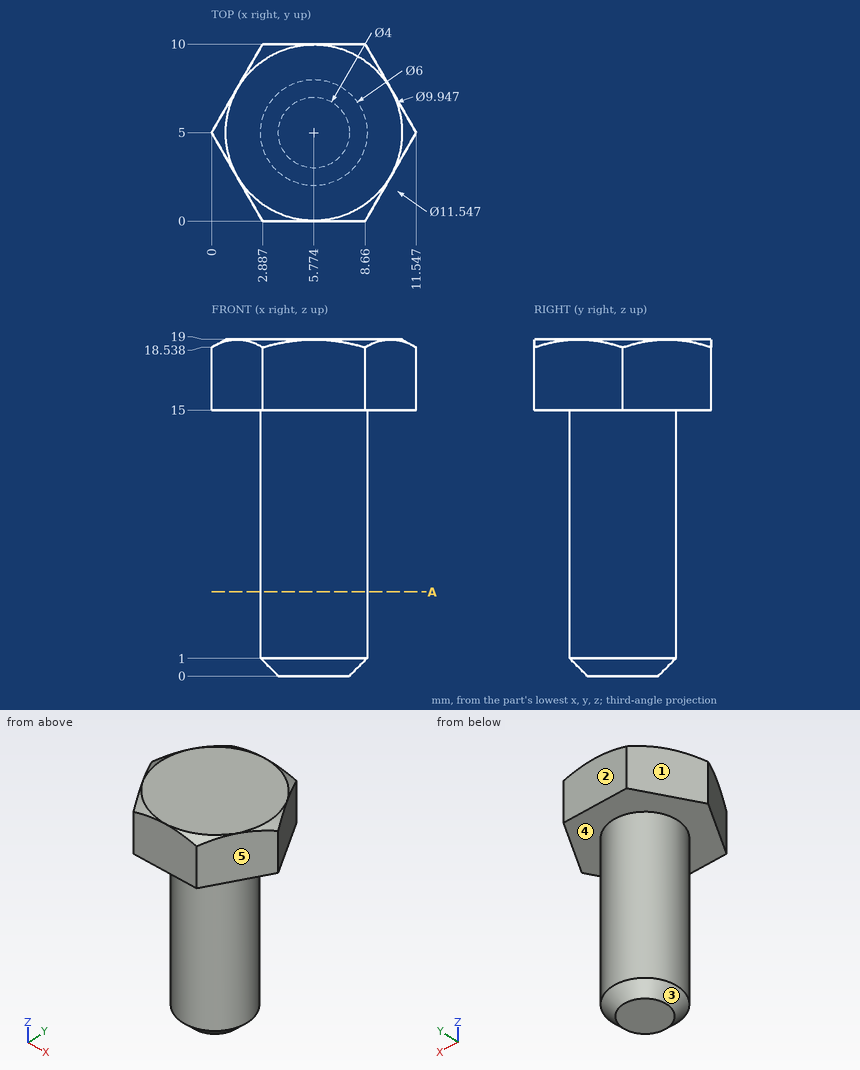
The figure shows three views and two pictorial views of one solid part (mm, origin at its lowest corner). Answer the questions. A direction names the side the tool comes from. Round coordinates to 2 decimals unless told otherwise and drop trailing zeros. Loops run counter-clockwise (first coordinate to the right, second up) from the corner with the lowest first, then second, coordinate; pieces in that order, holes last. Notation, with made-up numbers: M 85.5,-10 L 89.5,-10 A24 ccw 89.5,29 Z; hole C 14,70 d8. An arc over 180 degrees is marked long. Use CSV: the item, a comma, the result in double quotes.
Q1. Each of these flat-tipped pins is pushed along its axis until it touches: pin 1 (3 mm diameter, centred on y = 6, z = 3, fed in from -X); pin 2 (1 mm diameter, centred on y = 3.5, z = 8, fed in from -X) (1 decimal); pin 3 (5 mm diameter, centred on y = 7.5, z = 13.5, fed in from -X). Where does it stop, or does it pass through?
Determined:
pin 1,"x = 2.77"
pin 2,"x = 2.9"
pin 3,"x = 0.29"
Q2. A tool of negligible diameter and unlimited length cuts with its end or side. For the marked faces 4 and 5, from which of +Z, -Z, +X, -X, +Y, -Y can it reach the whole face along a straight path? Write none if from no direction.
Determined:
face 4,"-Z"
face 5,"+Z, -Z, +X, -Y"
Q3. Consider L1, parallel to Z at x = 1.5, y = 5.75; L2, parallel to X at y = 5, z = 5.75; L3, parallel to X at y = 5.5, z = 6 (1 decimal). Determine where each line is inside the solid, lowest interval first.
Determined:
L1,"15 to 19"
L2,"2.77 to 8.77"
L3,"2.8 to 8.7"
Q4. Section A-A, the plane z = 4.75 is taken. Determine the outline of the cut face in (x, y).
Determined:
outline,"C 5.77,5 d6"
Q5. The mould has two halves that part along X. Classify the marked faces 1, 2 and 3: pulls with the +X half, pulls with the -X half, needs draft (parallel to the pull), parting line crosses it, or undercut.
Determined:
face 1,"pulls with the -X half"
face 2,"needs draft"
face 3,"parting line crosses it"
